For this review, use the dimensioned drawing (mm, ordinates from the lowest corner) and the shaded views. A direction names the side the tool comes from. Coordinates: 2 decimals unless noted, no trailing zeros. Order: outer loops, then holes, each group sorted by start corner. A loop starts at its lowest first (then second) coordinate and runs counter-clockwise, first axis right, second up. Notation, with made-up numbers: M -29.5,-37 L -6.5,-37 A13 cw -6.5,-18 Z; hole C -39.75,-12.5 d10. An arc over 180 degrees is marked long. One line per item, written item: value.
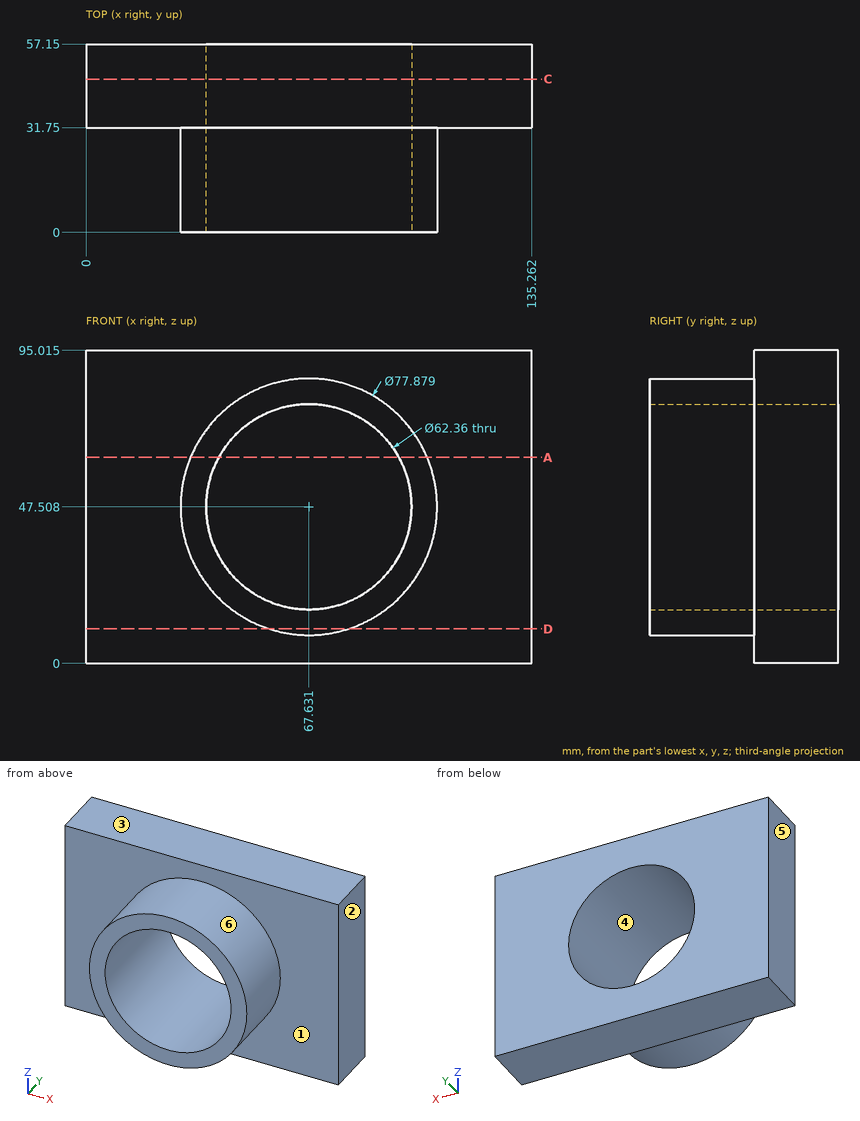
(1) We need section D-D, the plane z = 10.5. State the section outline as (x, y) points.
Geometry results:
outline: M 0,31.75 L 55.52,31.75 L 55.52,0 L 79.74,0 L 79.74,31.75 L 135.26,31.75 L 135.26,57.15 L 0,57.15 Z
(2) For L1, parallel to Y at x = 50.5, z = 83; L2, parallel to Z at x = 73, y = 44 (1 decimal); L3, parallel to X at y = 16, z = 19.5 (1 decimal), list the stretches that pass through material, from the lowest coordinate up.
Geometry results:
L1: y = 31.75 to 57.15
L2: z = 0 to 16.8, 78.2 to 95
L3: x = 40.6 to 53.9, 81.3 to 94.7
(3) Mouldability with a two-part tool opening along X and no side actions: class the marked faces 3, 4, 5 and 6 as +X half, -X half, draft (parallel to the pull), parting line (faces both ways), or undercut.
Geometry results:
face 3: draft
face 4: undercut
face 5: -X half
face 6: parting line
(4) We need section A-A, the plane z = 62.5. State the section outline as (x, y) points, plus the area to 3 significant figures.
Geometry results:
outline: M 0,31.75 L 31.69,31.75 L 31.69,0 L 40.29,0 L 40.29,57.15 L 0,57.15 Z; M 94.97,0 L 103.57,0 L 103.57,31.75 L 135.26,31.75 L 135.26,57.15 L 94.97,57.15 Z
area: 2,590 mm2
(5) Insertion check: pin 1 Ø1.5 at (y, z) = (22.5, 18) entering from +X (1 decimal); pin 2 Ø4 at (x, z) = (31, 54) entering from -Y; pin 3 Ø3 at (y, z) = (22, 62) entering from -X; pin 4 Ø4 at (y, z) = (12, 75) entering from -X (1 decimal). Each pin has a flat end and moves straight along its axis. Give the tip position at first contact, or say it passes through.
Geometry results:
pin 1: stops at x = 93.9
pin 2: stops at y = 0
pin 3: stops at x = 30.92
pin 4: stops at x = 38.2
(6) We need section C-C, the plane y = 46.5. State the section outline as (x, z) points (1 decimal), plus the area to 3 significant figures.
Geometry results:
outline: M 0,0 L 135.3,0 L 135.3,95 L 0,95 Z; hole C 67.6,47.5 d62.4
area: 9,800 mm2
(7) Tool access review of the marked faces 1 and 2: name each direction out of +Z, -Z, +X, -X, +Y, -Y from which nothing blocks a thin tool from reaching the whole face with its end or side.
Geometry results:
face 1: -Y
face 2: +Z, -Z, +X, +Y, -Y
